```python
from build123d import *

# Parameters (mm, degrees)
SKETCH2_W           = 200
SKETCH2_H           = 140
BOSS_EXTRUDE1_DEPTH = 6
FILLET1_R           = 5
SKETCH3_R           = 2.5
CUT_EXTRUDE1_DEPTH  = 123.21292894
SKETCH4_R           = 8
CUT_EXTRUDE2_DEPTH  = 123.21292894
CUT_EXTRUDE4_DEPTH  = 123.21292894
SKETCH7_R           = 2
CUT_EXTRUDE5_DEPTH  = 123.21292894


with BuildPart() as part:
    # Sketch2 → Boss-Extrude1 (new body)
    with BuildSketch(Plane(origin=(0, 0, 0), x_dir=(1, 0, 0), z_dir=(0, 1, 0))):
        Rectangle(SKETCH2_W, SKETCH2_H)
    extrude(amount=BOSS_EXTRUDE1_DEPTH)

    # Fillet1
    fillet1_edges = [part.edges().sort_by_distance(p)[0] for p in [
        (100, 3, 70),
        (-100, 3, 70),
        (-100, 3, -70),
        (100, 3, -70),
    ]]
    fillet(fillet1_edges, radius=FILLET1_R)

    # Sketch3 → Cut-Extrude1 (cut, through all)
    with BuildSketch(Plane(origin=(0, 6, 0), x_dir=(1, 0, 0), z_dir=(0, 1, 0))):
        with Locations(Location((-85, 55, 0), (0, 0, 270))):
            Circle(SKETCH3_R)
        with Locations(Location((-85, -55, 0), (0, 0, 90))):
            Circle(SKETCH3_R)
    extrude(amount=-CUT_EXTRUDE1_DEPTH, mode=Mode.SUBTRACT)

    # Sketch4 → Cut-Extrude2 (cut, through all)
    with BuildSketch(Plane(origin=(0, 6, 0), x_dir=(1, 0, 0), z_dir=(0, 1, 0))):
        with Locations(Location((0, 0, 0), (0, 0, 270))):
            Circle(SKETCH4_R)
    extrude(amount=-CUT_EXTRUDE2_DEPTH, mode=Mode.SUBTRACT)

    # Sketch6 → Cut-Extrude4 (cut, through all)
    with BuildSketch(Plane(origin=(0, 6, 0), x_dir=(1, 0, 0), z_dir=(0, 1, 0))):
        with BuildLine():
            Line((-74.688373307, 9.463724756), (-57.188373307, 9.463724756))
            ThreePointArc((-57.188373307, 9.463724756), (-54.938373307, 7.213724756), (-57.188373307, 4.963724756))
            Line((-57.188373307, 4.963724756), (-74.688373307, 4.963724756))
            ThreePointArc((-74.688373307, 4.963724756), (-76.938373307, 7.213724756), (-74.688373307, 9.463724756))
        make_face()
        with BuildLine():
            Line((-74.74772766, -4.486928349), (-57.24772766, -4.486928349))
            ThreePointArc((-57.24772766, -4.486928349), (-54.99772766, -6.736928349), (-57.24772766, -8.986928349))
            Line((-57.24772766, -8.986928349), (-74.74772766, -8.986928349))
            ThreePointArc((-74.74772766, -8.986928349), (-76.99772766, -6.736928349), (-74.74772766, -4.486928349))
        make_face()
    extrude(amount=-CUT_EXTRUDE4_DEPTH, mode=Mode.SUBTRACT)

    # Sketch7 → Cut-Extrude5 (cut, through all)
    with BuildSketch(Plane(origin=(0, 6, 0), x_dir=(1, 0, 0), z_dir=(0, 1, 0))):
        with Locations(Location((42.902668062, -32.720520695, 0), (0, 0, 270))):
            Circle(SKETCH7_R)
        with Locations(Location((42.902668062, 34.418343412, 0), (0, 0, 270))):
            Circle(SKETCH7_R)
    extrude(amount=-CUT_EXTRUDE5_DEPTH, mode=Mode.SUBTRACT)


solid = part.part
```
Read the model definition and answer for the solid it produces. Units are mm, in the model's axes. A direction names the side the tool comes from. Round coordinates to 2 decimals unless told otherwise and drop trailing zeros. Write each loop counter-clockwise with the first axis right and the second up, starting at its lowest first coordinate (ties: lowest second). Pieces come first, ordered by that corner, then holes. Notation, with made-up numbers: (-11.75, 7.25) - (-5.75, 7.25) arc R22 ccw to (-5.75, 38.25) - close; hole circle Ø3 at (31.5, 46). An arc over 180 degrees is marked (long way). Use CSV: the item, a comma, the result in double quotes.
Q1. A tool of negligible diameter and unlimited length cuts with its end or side. For faces 5 (the flat face through (-66, 3, -4.964)), 6 (the cylindrical face through (-99, 3, 68)), from which of +Z, -Z, +X, -X, +Y, -Y can it reach the whole face along a straight path? Write none if from no direction.
Values:
face 5,"+Y, -Y"
face 6,"+Z, -X, +Y, -Y"
Q2. Find section C-C, the plane x = -85. Write down the section's boundary in (y, z), then the cut area to 3 significant figures.
Values:
outline,"(0, -70) - (6, -70) - (6, -57.5) - (0, -57.5) - close; (0, -52.5) - (6, -52.5) - (6, 52.5) - (0, 52.5) - close; (0, 57.5) - (6, 57.5) - (6, 70) - (0, 70) - close"
area,"780 mm²"
Q3. Find section D-D, the plane y = 3.75. Write down the section's boundary in (x, z), then the cut area to 3 significant figures.
Values:
outline,"(-100, -65) arc R5 ccw to (-95, -70) - (95, -70) arc R5 ccw to (100, -65) - (100, 65) arc R5 ccw to (95, 70) - (-95, 70) arc R5 ccw to (-100, 65) - close; hole circle Ø5 at (-85, -55); hole circle Ø5 at (-85, 55); hole (-74.75, 4.49) - (-57.25, 4.49) arc R2.25 ccw to (-57.25, 8.99) - (-74.75, 8.99) arc R2.25 ccw to start; hole (-74.69, -9.46) - (-57.19, -9.46) arc R2.25 ccw to (-57.19, -4.96) - (-74.69, -4.96) arc R2.25 ccw to start; hole circle Ø16 at (0, 0); hole circle Ø4 at (42.9, -34.42); hole circle Ø4 at (42.9, 32.72)"
area,"27,500 mm²"
Q4. Determine the mould class of faces 1 (the cylindrical face through (-76.938, 3.042, -7.164)), 2 (the flat face through (-1, 3, 70)), 3 (the cylindrical face through (-76.997, 3.042, 6.786)), 4 (the flat face through (-100, 3, 1)) for opening direction Z: +Z half, -Z half, draft (parallel to the pull), parting line (faces both ways), or undercut.
Values:
face 1,"undercut"
face 2,"+Z half"
face 3,"undercut"
face 4,"draft"
Q5. Find section B-B, the plane z = 55. Write down the section's boundary in (x, y), then the cut area to 3 significant figures.
Values:
outline,"(-100, 0) - (-87.5, 0) - (-87.5, 6) - (-100, 6) - close; (-82.5, 0) - (100, 0) - (100, 6) - (-82.5, 6) - close"
area,"1,170 mm²"
Q6. Straight lines are drawn through the part: line 1 along Z through (x, y) = (-62, 1.7); line 2 along X through (y, z) = (2.05, 0); line 3 along X through (y, z) = (3.95, 55). For each, find the intervals that lie inside material, in ascending order.
Values:
line 1,"z = -70 to -9.46, -4.96 to 4.49, 8.99 to 70"
line 2,"x = -100 to -8, 8 to 100"
line 3,"x = -100 to -87.5, -82.5 to 100"
Q7. Find section A-A, the plane x = 0. Write down the section's boundary in (y, z).
Values:
outline,"(0, -70) - (6, -70) - (6, -8) - (0, -8) - close; (0, 8) - (6, 8) - (6, 70) - (0, 70) - close"
